CAD build for the part. Positions are in the model's coordinates, mm. A direction names the side the tool comes from. Give positions to 0.01 mm unless a question says otherwise; leave off trailing zeros. Write each loop counter-clockwise with the first axis right and the second up, starting at its lowest first coordinate (ties: lowest second). Pieces come first, ordered by that corner, then holes. Notation, with made-up numbers: (-29.5, 38.25) -> (23.5, 38.25) arc R20 ccw to (23.5, 69.25) -> close; hole circle Ø2 at (-21.75, -24.5). An arc over 180 degrees is marked (long way). Answer in a Markdown table with one row per item. Add a question column.
```python
from build123d import *

# Parameters (mm, degrees)
SKETCH1_W                 = 12.573
SKETCH1_H                 = 12.573
SKETCH1_W_2               = 11.557
SKETCH1_H_2               = 11.557
EXTRUDE_THIN1_DEPTH       = 6.35
SKETCH1_4_W               = 12.573
SKETCH1_4_H               = 0.508
EXTRUDE_THIN2_DEPTH       = 6.35
SKETCH2_W                 = 14.097
SKETCH2_H                 = 14.097
SKETCH2_W_2               = 12.573
SKETCH2_H_2               = 12.573
BOSS_EXTRUDE1_DEPTH       = 3.175
SKETCH3_R                 = 1.27
BOSS_EXTRUDE2_DEPTH       = 3.175
FILLET2_R                 = 1.27
CHAMFER1_SIZE             = 0.508
F_0_80_TAPPED_HOLE1_D     = 1.19126
F_0_80_TAPPED_HOLE1_DEPTH = 3.302
F_0_80_TAPPED_HOLE1_TIP   = 0.357890611
SKETCH6_W                 = 1.27
SKETCH6_H                 = 1.27
EXTRUDE_THIN3_DEPTH       = 1.5875
CHAMFER2_SIZE             = 0.254


with BuildPart() as part:
    # Sketch1 → Extrude-Thin1 (new body)
    with BuildSketch(Plane.XY):
        with Locations((-12.7, -106.3625)):
            Rectangle(SKETCH1_W, SKETCH1_H)
        with Locations((-12.7, -106.3625)):
            Rectangle(SKETCH1_W_2, SKETCH1_H_2, mode=Mode.SUBTRACT)
    extrude(amount=EXTRUDE_THIN1_DEPTH)

    # Sketch1<4> → Extrude-Thin2 (add, through all)
    with BuildSketch(Plane.XY):
        with Locations((-12.7, -106.3625)):
            Rectangle(SKETCH1_4_W, SKETCH1_4_H)
    extrude(amount=EXTRUDE_THIN2_DEPTH)

    # Sketch2 → Boss-Extrude1 (add)
    with BuildSketch(Plane.XY.offset(6.35)):
        with Locations((-12.7, -106.3625)):
            Rectangle(SKETCH2_W, SKETCH2_H)
        with Locations((-12.7, -106.3625)):
            Rectangle(SKETCH2_W_2, SKETCH2_H_2, mode=Mode.SUBTRACT)
    extrude(amount=-BOSS_EXTRUDE1_DEPTH)

    # Sketch3 → Boss-Extrude2 (add)
    with BuildSketch(Plane.XY.offset(6.35)):
        with Locations((-12.7, -106.3625)):
            Circle(SKETCH3_R)
    extrude(amount=-BOSS_EXTRUDE2_DEPTH)

    # Fillet2
    fillet2_edges = [part.edges().sort_by_distance(p)[0] for p in [
        (-13.944340789, -106.6165, 4.7625),
        (-11.455659211, -106.6165, 4.7625),
        (-11.455659211, -106.1085, 4.7625),
        (-13.944340789, -106.1085, 4.7625),
    ]]
    fillet(fillet2_edges, radius=FILLET2_R)

    # Chamfer1
    chamfer1_edges = [part.edges().sort_by_distance(p)[0] for p in [
        (-12.7, -106.6165, 3.175),
        (-12.7, -106.1085, 3.175),
    ]]
    chamfer(chamfer1_edges, length=CHAMFER1_SIZE)

    # #0-80 Tapped Hole1
    with Locations(Plane.XY.offset(6.35)):
        with Locations((-12.7, -106.3625)):
            Hole(F_0_80_TAPPED_HOLE1_D / 2, depth=F_0_80_TAPPED_HOLE1_DEPTH)
            with Locations((0, 0, -(F_0_80_TAPPED_HOLE1_DEPTH + F_0_80_TAPPED_HOLE1_TIP / 2))):  # 118° drill point
                Cone(0, F_0_80_TAPPED_HOLE1_D / 2, F_0_80_TAPPED_HOLE1_TIP, mode=Mode.SUBTRACT)

    # Sketch6 → Extrude-Thin3 (add)
    with BuildSketch(Plane.XY.offset(6.35)):
        with Locations((-12.7, -114.046)):
            Rectangle(SKETCH6_W, SKETCH6_H)
        with Locations((-9.17575, -98.679)):
            Rectangle(SKETCH6_W, SKETCH6_H)
        with Locations((-16.22425, -98.679)):
            Rectangle(SKETCH6_W, SKETCH6_H)
    extrude(amount=-EXTRUDE_THIN3_DEPTH)

    # Chamfer2
    chamfer2_edges = [part.edges().sort_by_distance(p)[0] for p in [
        (-12.7, -114.681, 4.7625),
        (-12.065, -114.046, 4.7625),
        (-13.335, -114.046, 4.7625),
        (-8.54075, -98.044, 5.55625),
        (-9.81075, -98.044, 5.55625),
        (-16.85925, -98.044, 5.55625),
        (-15.58925, -98.044, 5.55625),
        (-13.335, -114.681, 5.55625),
        (-12.065, -114.681, 5.55625),
        (-9.81075, -98.679, 4.7625),
        (-8.54075, -98.679, 4.7625),
        (-9.17575, -98.044, 4.7625),
        (-16.85925, -98.679, 4.7625),
        (-16.22425, -98.044, 4.7625),
        (-15.58925, -98.679, 4.7625),
    ]]
    chamfer(chamfer2_edges, length=CHAMFER2_SIZE)


solid = part.part
```
Item 1: Drop flat-ended pins along their axis: pin 1 Ø3.5 at (x, z) = (-11.5, 5) entering from -Y; pin 2 Ø3 at (x, z) = (-10, 3.5) entering from -Y; pin 3 Ø0.8 at (y, z) = (-98.5, 6) entering from +X; pin 4 Ø1.7 at (y, z) = (-109.5, 1.5) entering from +X. Give the stop position or say it passes through.
Item 2: Probe L1, parallel to Y at x = -12.7, z = 5.05; L2, parallel to Y at x = -7.75, z = 1.25; L3, parallel to Y at x = -12.7, z = 4. List the from-to ranges inside material, lowest first. Write a range as from..to.
Item 3: Slice it at B-B, the plane z = 0.5. List the corners of the cut face in (x, y), then the cut area to 3 significant figures.
Item 4: Which spindle directions (+Z, -Z, +X, -X, +Y, -Y) get a long thin tool onto all of the face, cutting with end or side? Do faces 5 (the face through (-15.589, -99, 6)), 6 (the face through (-12.571, -106.944, 4.676)), 7 (the face through (-6.921, -109, 3)), 8 (the face through (-8.541, -99, 6)), 9 (the face through (-13, -106.616, 2)). Say none if no direction does.
Item 5: Mould opens along X. For faces 1 (the face through (-13, -100.076, 2)), 2 (the face through (-13, -99.314, 5)), 3 (the face through (-6.413, -106, 2)), 4 (the face through (-19.748, -106, 5)) say: released by +X, released by -X, zero draft, split by the parting line, or undercut.
Item 6: Slice it at A-A, the plane x = -16.25. State how many separate pieces and enclosed holes the cut face has, then the cut area to 3 significant figures.
Item 7: Slice it at C-C, the plane z = 4.5. List the corners of the cut face in (x, y).
Answer key:
| question | item | result |
|---|---|---|
| 1 | pin 1 | stops at y = -114.68 |
| 1 | pin 2 | stops at y = -113.41 |
| 1 | pin 3 | stops at x = -8.54 |
| 1 | pin 4 | stops at x = -6.41 |
| 2 | L1 | y = -114.68..-112.14, -107.63..-106.96, -105.77..-105.09, -100.58..-99.31 |
| 2 | L2 | y = -112.65..-112.14, -106.62..-106.11, -100.58..-100.08 |
| 2 | L3 | y = -113.41..-112.14, -107.63..-106.96, -105.77..-105.09, -100.58..-99.31 |
| 3 | outline | (-18.99, -112.65) -> (-6.41, -112.65) -> (-6.41, -100.08) -> (-18.99, -100.08) -> close; hole (-18.48, -112.14) -> (-6.92, -112.14) -> (-6.92, -106.62) -> (-18.48, -106.62) -> close; hole (-18.48, -106.11) -> (-6.92, -106.11) -> (-6.92, -100.58) -> (-18.48, -100.58) -> close |
| 3 | area | 30.4 mm² |
| 4 | face 5 | +Z, -Z, +Y |
| 4 | face 6 | +Z |
| 4 | face 7 | +Z, -Z |
| 4 | face 8 | +Z, -Z, +X, +Y |
| 4 | face 9 | -Z |
| 5 | face 1 | zero draft |
| 5 | face 2 | undercut |
| 5 | face 3 | released by +X |
| 5 | face 4 | released by -X |
| 6 | separate pieces | 3 |
| 6 | enclosed holes | 0 |
| 6 | area | 16.5 mm² |
| 7 | outline | (-19.75, -113.41) -> (-5.65, -113.41) -> (-5.65, -99.31) -> (-19.75, -99.31) -> close; hole (-18.48, -112.14) -> (-6.92, -112.14) -> (-6.92, -106.62) -> (-10.67, -106.62) arc R1.27 ccw to (-11.68, -107.12) arc R1.27 cw to (-13.72, -107.12) arc R1.27 ccw to (-14.73, -106.62) -> (-18.48, -106.62) -> close; hole (-18.48, -106.11) -> (-14.73, -106.11) arc R1.27 ccw to (-13.72, -105.6) arc R1.27 cw to (-11.68, -105.6) arc R1.27 ccw to (-10.67, -106.11) -> (-6.92, -106.11) -> (-6.92, -100.58) -> (-18.48, -100.58) -> close; hole circle Ø1.19 at (-12.7, -106.36) |
